```python
from build123d import *

# Parameters (mm, degrees)
BOSS_EXTRUDE1_DEPTH = 8


with BuildPart() as part:
    # Sketch1 → Boss-Extrude1 (new body)
    with BuildSketch(Plane(origin=(0, 0, 0), x_dir=(1, 0, 0), z_dir=(0, 1, 0))):
        with BuildLine():
            ThreePointArc((5.756768163, 29.44247986), (4.693033951, 29.630650218), (3.62321476, 29.780401522))
            Line((3.62321476, 29.780401522), (1.299038106, 25.754809472))
            ThreePointArc((1.299038106, 25.754809472), (0, 25.004809472), (-1.299038106, 25.754809472))
            Line((-1.299038106, 25.754809472), (-3.62321476, 29.780401522))
            ThreePointArc((-3.62321476, 29.780401522), (-4.693033951, 29.630650218), (-5.756768163, 29.44247986))
            Line((-5.756768163, 29.44247986), (-6.723215158, 24.895704225))
            ThreePointArc((-6.723215158, 24.895704225), (-7.726911068, 23.780986987), (-9.194132469, 24.092854523))
            Line((-9.194132469, 24.092854523), (-12.648532177, 27.20320999))
            ThreePointArc((-12.648532177, 27.20320999), (-13.619714992, 26.730195726), (-14.573238507, 26.222523132))
            Line((-14.573238507, 26.222523132), (-14.087353279, 21.59963399))
            ThreePointArc((-14.087353279, 21.59963399), (-14.697458244, 20.229315804), (-16.189241087, 20.072523109))
            Line((-16.189241087, 20.072523109), (-20.435723137, 21.963178729))
            ThreePointArc((-20.435723137, 21.963178729), (-21.213203436, 21.213203436), (-21.963178729, 20.435723137))
            Line((-21.963178729, 20.435723137), (-20.072523109, 16.189241087))
            ThreePointArc((-20.072523109, 16.189241087), (-20.229315804, 14.697458244), (-21.59963399, 14.087353279))
            Line((-21.59963399, 14.087353279), (-26.222523132, 14.573238507))
            ThreePointArc((-26.222523132, 14.573238507), (-26.730195726, 13.619714992), (-27.20320999, 12.648532177))
            Line((-27.20320999, 12.648532177), (-24.092854523, 9.194132469))
            ThreePointArc((-24.092854523, 9.194132469), (-23.780986987, 7.726911068), (-24.895704225, 6.723215158))
            Line((-24.895704225, 6.723215158), (-29.44247986, 5.756768163))
            ThreePointArc((-29.44247986, 5.756768163), (-29.630650218, 4.693033951), (-29.780401522, 3.62321476))
            Line((-29.780401522, 3.62321476), (-25.754809472, 1.299038106))
            ThreePointArc((-25.754809472, 1.299038106), (-25.004809472, 0), (-25.754809472, -1.299038106))
            Line((-25.754809472, -1.299038106), (-29.780401522, -3.62321476))
            ThreePointArc((-29.780401522, -3.62321476), (-29.630650218, -4.693033951), (-29.44247986, -5.756768163))
            Line((-29.44247986, -5.756768163), (-24.895704225, -6.723215158))
            ThreePointArc((-24.895704225, -6.723215158), (-23.780986987, -7.726911068), (-24.092854523, -9.194132469))
            Line((-24.092854523, -9.194132469), (-27.20320999, -12.648532177))
            ThreePointArc((-27.20320999, -12.648532177), (-26.730195726, -13.619714992), (-26.222523132, -14.573238507))
            Line((-26.222523132, -14.573238507), (-21.59963399, -14.087353279))
            ThreePointArc((-21.59963399, -14.087353279), (-20.229315804, -14.697458244), (-20.072523109, -16.189241087))
            Line((-20.072523109, -16.189241087), (-21.963178729, -20.435723137))
            ThreePointArc((-21.963178729, -20.435723137), (-21.213203436, -21.213203436), (-20.435723137, -21.963178729))
            Line((-20.435723137, -21.963178729), (-16.189241087, -20.072523109))
            ThreePointArc((-16.189241087, -20.072523109), (-14.697458244, -20.229315804), (-14.087353279, -21.59963399))
            Line((-14.087353279, -21.59963399), (-14.573238507, -26.222523132))
            ThreePointArc((-14.573238507, -26.222523132), (-13.619714992, -26.730195726), (-12.648532177, -27.20320999))
            Line((-12.648532177, -27.20320999), (-9.194132469, -24.092854523))
            ThreePointArc((-9.194132469, -24.092854523), (-7.726911068, -23.780986987), (-6.723215158, -24.895704225))
            Line((-6.723215158, -24.895704225), (-5.756768163, -29.44247986))
            ThreePointArc((-5.756768163, -29.44247986), (-4.693033951, -29.630650218), (-3.62321476, -29.780401522))
            Line((-3.62321476, -29.780401522), (-1.299038106, -25.754809472))
            ThreePointArc((-1.299038106, -25.754809472), (0, -25.004809472), (1.299038106, -25.754809472))
            Line((1.299038106, -25.754809472), (3.62321476, -29.780401522))
            ThreePointArc((3.62321476, -29.780401522), (4.693033951, -29.630650218), (5.756768163, -29.44247986))
            Line((5.756768163, -29.44247986), (6.723215158, -24.895704225))
            ThreePointArc((6.723215158, -24.895704225), (7.726911068, -23.780986987), (9.194132469, -24.092854523))
            Line((9.194132469, -24.092854523), (12.648532177, -27.20320999))
            ThreePointArc((12.648532177, -27.20320999), (13.619714992, -26.730195726), (14.573238507, -26.222523132))
            Line((14.573238507, -26.222523132), (14.087353279, -21.59963399))
            ThreePointArc((14.087353279, -21.59963399), (14.697458244, -20.229315804), (16.189241087, -20.072523109))
            Line((16.189241087, -20.072523109), (20.435723137, -21.963178729))
            ThreePointArc((20.435723137, -21.963178729), (21.213203436, -21.213203436), (21.963178729, -20.435723137))
            Line((21.963178729, -20.435723137), (20.072523109, -16.189241087))
            ThreePointArc((20.072523109, -16.189241087), (20.229315804, -14.697458244), (21.59963399, -14.087353279))
            Line((21.59963399, -14.087353279), (26.222523132, -14.573238507))
            ThreePointArc((26.222523132, -14.573238507), (26.730195726, -13.619714992), (27.20320999, -12.648532177))
            Line((27.20320999, -12.648532177), (24.092854523, -9.194132469))
            ThreePointArc((24.092854523, -9.194132469), (23.780986987, -7.726911068), (24.895704225, -6.723215158))
            Line((24.895704225, -6.723215158), (29.44247986, -5.756768163))
            ThreePointArc((29.44247986, -5.756768163), (29.630650218, -4.693033951), (29.780401522, -3.62321476))
            Line((29.780401522, -3.62321476), (25.754809472, -1.299038106))
            ThreePointArc((25.754809472, -1.299038106), (25.004809472, 0), (25.754809472, 1.299038106))
            Line((25.754809472, 1.299038106), (29.780401522, 3.62321476))
            ThreePointArc((29.780401522, 3.62321476), (29.630650218, 4.693033951), (29.44247986, 5.756768163))
            Line((29.44247986, 5.756768163), (24.895704225, 6.723215158))
            ThreePointArc((24.895704225, 6.723215158), (23.780986987, 7.726911068), (24.092854523, 9.194132469))
            Line((24.092854523, 9.194132469), (27.20320999, 12.648532177))
            ThreePointArc((27.20320999, 12.648532177), (26.730195726, 13.619714992), (26.222523132, 14.573238507))
            Line((26.222523132, 14.573238507), (21.59963399, 14.087353279))
            ThreePointArc((21.59963399, 14.087353279), (20.229315804, 14.697458244), (20.072523109, 16.189241087))
            Line((20.072523109, 16.189241087), (21.963178729, 20.435723137))
            ThreePointArc((21.963178729, 20.435723137), (21.213203436, 21.213203436), (20.435723137, 21.963178729))
            Line((20.435723137, 21.963178729), (16.189241087, 20.072523109))
            ThreePointArc((16.189241087, 20.072523109), (14.697458244, 20.229315804), (14.087353279, 21.59963399))
            Line((14.087353279, 21.59963399), (14.573238507, 26.222523132))
            ThreePointArc((14.573238507, 26.222523132), (13.619714992, 26.730195726), (12.648532177, 27.20320999))
            Line((12.648532177, 27.20320999), (9.194132469, 24.092854523))
            ThreePointArc((9.194132469, 24.092854523), (7.726911068, 23.780986987), (6.723215158, 24.895704225))
            Line((6.723215158, 24.895704225), (5.756768163, 29.44247986))
        make_face()
        with BuildLine():
            ThreePointArc((5, 0), (-3.061862178, -3.952847075), (-1.25, 4.841229183))
            Line((-1.25, 4.841229183), (-1.25, 7))
            Line((-1.25, 7), (1.25, 7))
            Line((1.25, 7), (1.25, 4.841229183))
            ThreePointArc((1.25, 4.841229183), (3.952847075, 3.061862178), (5, 0))
        make_face(mode=Mode.SUBTRACT)
    extrude(amount=BOSS_EXTRUDE1_DEPTH)


solid = part.part
```
Design review of the part built by this model. Coordinates are the model's own, in mm. A direction names the side the tool comes from. Coordinates: 2 decimals unless noted, no trailing zeros. Order: outer loops, then holes, each group sorted by start corner. A loop starts at its lowest first (then second) coordinate and runs counter-clockwise, first axis right, second up.
1) Clearance check with flat-ended pins moving along their axes: pin 1 (4 mm diameter, centred on x = 9, y = 3.5, fed in from -Z); pin 2 (0.6 mm diameter, centred on y = 3, z = -6, fed in from +X); pin 3 (8 mm diameter, centred on x = -22, z = -16.5, fed in from +Y); pin 4 (3 mm diameter, centred on x = -14, y = 5, fed in from +Z). State where each tip first meets the part, or that it passes through.
2) Take a section at A-A, the plane x = 0. Give the boundary of the cut face in (y, z).
3) Wall thickness on line 1 along X through (y, z) = (5.75, 27); line 2 along X through (y, z) = (7, -24); line 3 along X through (y, z) = (3.5, -17): over which ranges is each line inside the solid? List them lowest first.
4) Take a section at B-B, the plane x = 11. Give the boundary of the cut face in (y, z), and give its area (3 significant figures).
5) Mouldability with a two-part tool opening along Z and no side actions: class faces 5 (the cylindrical face through (-26.737, 3.944, 13.606)), 6 (the flat face through (-27.137, 3.944, -6.247)), 7 (the flat face through (-6.233, 3.944, -27.201)), 8 (the flat face through (-21.005, 3.944, 18.283)) as +Z half, -Z half, draft (parallel to the pull), parting line (faces both ways), or undercut.
6) For faces 1 (the flat face through (-10.9, 3.94, -25.63)), 2 (the flat face through (-25.63, 3.94, 10.9)), 3 (the flat face through (27.137, 3.944, 6.247)), 4 (the cylindrical face through (20.217, 3.944, 14.715)), list the 3-axis set-ups (+Z, -Z, +X, -X, +Y, -Y) from which the entire face can be reached by the end or side of a thin tool; tool diameter is ignored.
7) Take a section at C-C, the plane z = 8. Give the boundary of the cut face in (x, y), and give its area (3 significant figures).
Returned:
1. pin 1: stops at z = -25.72
1. pin 2: stops at x = 29.45
1. pin 3: stops at y = 8
1. pin 4: stops at z = 27.2
2. outline: (0, -25) - (8, -25) - (8, -7) - (0, -7) - close; (0, 5) - (8, 5) - (8, 25) - (0, 25) - close
3. line 1: x = -13.08 to -12.42, -6.28 to -2.02, 2.02 to 6.28, 12.42 to 13.08
3. line 2: x = -14.34 to -9.08, -7.3 to 7.3, 9.08 to 14.34
3. line 3: x = -20.43 to 20.43
4. outline: (0, -25.72) - (8, -25.72) - (8, 25.72) - (0, 25.72) - close
4. area: 412 mm2
5. face 5: +Z half
5. face 6: undercut
5. face 7: -Z half
5. face 8: undercut
6. face 1: -Z, +Y, -Y
6. face 2: -X, +Y, -Y
6. face 3: +X, +Y, -Y
6. face 4: +Y, -Y
7. outline: (-23.72, 0) - (23.72, 0) - (23.72, 8) - (-23.72, 8) - close
7. area: 380 mm2
